Design review of the part shown in the three views and the two pictorial views. Dimensions are in mm from the part's minimum x, y and z. A direction names the side the tool comes from. Give positions to 0.01 mm unless a question says otherwise; leave off trailing zeros. Order: outer loops, then holes, each group sorted by start corner. A loop starts at its lowest first (then second) coordinate and runs counter-clockwise, first axis right, second up.
Item 1: Consider section D-D (y = 5.5). Give the boundary of the cut face in (x, z), plus the area to 3 significant figures.
Item 2: Consider section B-B (y = 16.5). Give the boundary of the cut face in (x, z), plus the area to 3 significant figures.
Item 3: Consider section C-C (x = 23.5). Give the boundary of the cut face in (y, z) (1 decimal).
Item 4: Machinability: for the marked faces 1, 2 and 3, which of the approach directions +Z, -Z, +X, -X, +Y, -Y give a long, thin tool a straight path to every point of the face, cutting with its end or side? Answer none if there is none.
Item 5: The part is to be moulded in two halves that separate along X. For the marked faces 4, 5 and 6, say which applies: released by +X, released by -X, zero draft, split by the parting line, or undercut.
Item 6: For probe 1 along Y at (x, z) = (25, 11.1); probe 2 along Z at (x, y) = (17, 17.5); probe 3 along Y at (x, z) = (25, 8.6), list the stretches that pass through material, from the lowest coordinate up.
Item 7: Consider section A-A (z = 6.75). Give the boundary of the cut face in (x, y), plus the area to 3 significant figures.
Item 8: For P1, Ø6, axis at y = 20.5, z = 3, coming from the +X side (3 decimals); P2, Ø3, axis at x = 31.5, y = 15.5, coming from the -Z side; P3, Ø3, axis at x = 9, z = 16, coming from the +Y side, all flat-tipped, find the tip position at first contact; note any pin that passes through.
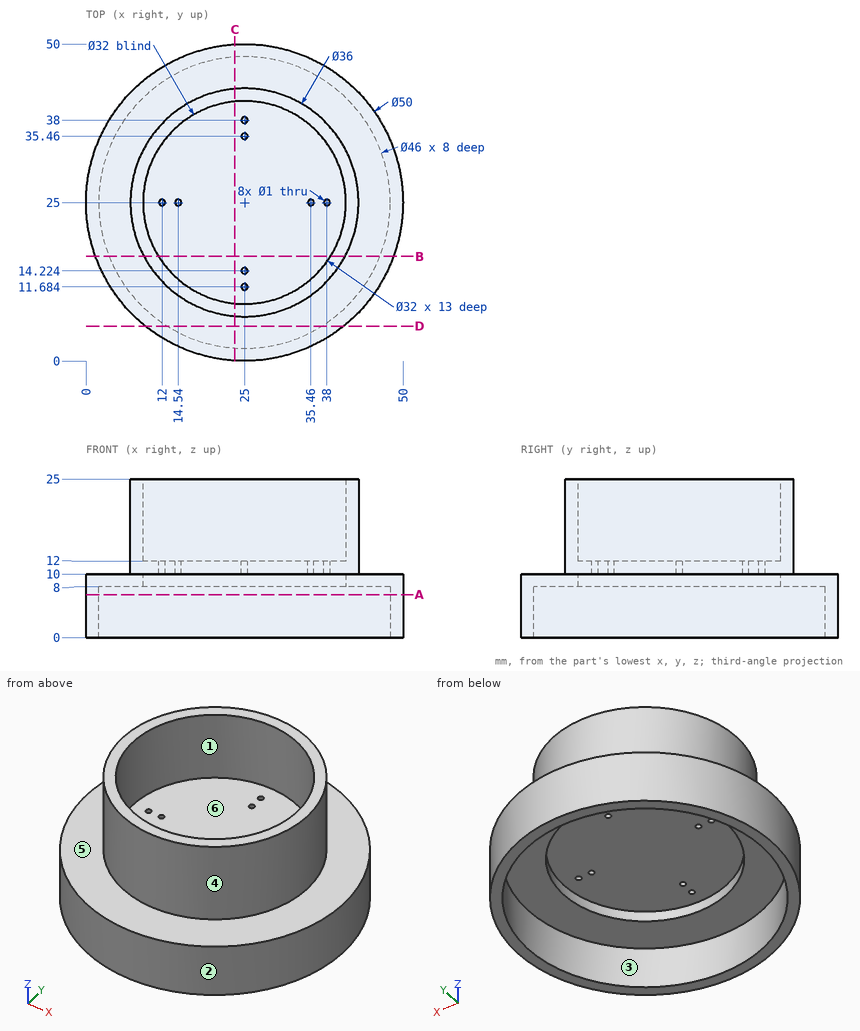
Resolved:
1. outline: (9.36, 0) - (12.8, 0) - (12.8, 8) - (37.2, 8) - (37.2, 0) - (40.64, 0) - (40.64, 10) - (9.36, 10) - close
1. area: 118 mm2
2. outline: (1.49, 0) - (3.63, 0) - (3.63, 8) - (11.44, 8) - (11.44, 10) - (38.56, 10) - (38.56, 8) - (46.37, 8) - (46.37, 0) - (48.51, 0) - (48.51, 10) - (40.87, 10) - (40.87, 25) - (38.56, 25) - (38.56, 12) - (11.44, 12) - (11.44, 25) - (9.13, 25) - (9.13, 10) - (1.49, 10) - close
2. area: 198 mm2
3. outline: (0, 0) - (2, 0) - (2, 8) - (9.1, 8) - (9.1, 10) - (40.9, 10) - (40.9, 8) - (48, 8) - (48, 0) - (50, 0) - (50, 10) - (42.9, 10) - (42.9, 25) - (40.9, 25) - (40.9, 12) - (9.1, 12) - (9.1, 25) - (7.1, 25) - (7.1, 10) - (0, 10) - close
4. face 1: +Z
4. face 2: +Z, -Z
4. face 3: -Z
5. face 4: split by the parting line
5. face 5: zero draft
5. face 6: undercut
6. probe 1: y = 7 to 11.18, 12.18 to 13.72, 14.72 to 34.96, 35.96 to 37.5, 38.5 to 43
6. probe 2: z = 10 to 12
6. probe 3: y = 0 to 9, 41 to 50
7. outline: circle Ø50 at (25, 25); hole circle Ø46 at (25, 25)
7. area: 302 mm2
8. P1: stops at x = 49.955
8. P2: stops at z = 10
8. P3: stops at y = 35.67
